Geometry: final body of the model. Coordinates: model frame, mm. A direction names the side the tool comes from. Give positions to 0.01 mm unless a question says otherwise; leave off trailing zeros. Write each loop counter-clockwise with the first axis right and the second up, starting at its lowest first coordinate (ties: lowest second). Pieces come first, ordered by that corner, then holes.
Q1. Section B-B (x = -60). Return the cut outline in (y, z), plus the area to 3 significant figures.
Q2. Section C-C (y = 41). Return the cut outline in (x, z).
Q3. Line query: line 1 (X direction, y = 33.5, z = 1); line 2 (X direction, y = 45.5, z = 9.5); line 3 (X direction, y = 41, z = 9.5). Output: solid intervals per line, ascending.
Q4. Pin query (flat end, axial travel): pin 1 Ø0.6 at (x, z) = (-8.5, 3.5) entering from -Y; pin 2 Ø1.1 at (x, z) = (-26, 4.5) entering from -Y; pin 3 Ø6 at (y, z) = (21.5, 2) entering from +X; pin 4 Ø1 at (x, y) = (-49, 39.5) entering from -Z. Return the tip coordinate at first contact, or that it passes through.
Q5. Section A-A (y = 26). State how many separate pieces and enclosed holes the cut face has, plus the area to 3 significant figures.
Q6. Reachability of faces 4 (the flat face through (-8.34, 38.96, 4.93)), 5 (the flat face through (-24.872, 44, 5)), 6 (the flat face through (-34, 34, 10)) from +Z, -Z, +X, -X, +Y, -Y: full face, straight path, thin tool, end or side. Return the list, or none.
Q7. Mould query, pull axis X, two halves, no side actions, for faces 1 (the cylindrical face through (-44.29, 23.48, 4.93)), 2 (the flat face through (-6.354, 38.929, 4.93)), 3 (the flat face through (-64.68, 48.8, 4.93)). Classes: +X half, -X half, draft (parallel to the pull), parting line (faces both ways), or undercut.
from build123d import *

# Parameters (mm, degrees)
F1_DEPTH = 10


with BuildPart() as f1:
    # F0 (on Top) → F1 (new body)
    with BuildSketch(Plane.XY):
        with BuildLine():
            ThreePointArc((-54.1309299153, 34.7543450507), (-54.1309291616, 34.7521602069), (-54.1309289103, 34.749975363))
            ThreePointArc((-54.1309289103, 34.749975363), (-54.1384443348, 34.3721704089), (-54.1609787174, 33.9949632158))
            ThreePointArc((-54.1609787174, 33.9949632158), (-54.0660685748, 32.5507467457), (-53.7734610387, 31.1333018692))
            ThreePointArc((-53.7734610387, 31.1333018692), (-53.3697669437, 32.5231940325), (-53.1610367081, 33.9553954277))
            ThreePointArc((-53.1610367081, 33.9553954277), (-53.1536089265, 34.335386944), (-53.130987906, 34.7147772626))
            ThreePointArc((-53.130987906, 34.7147772626), (-53.1309436593, 34.7323762881), (-53.1309289103, 34.749975363))
            ThreePointArc((-53.1309289103, 34.749975363), (-53.2282743232, 36.1764316505), (-53.5185055847, 37.5764386092))
            ThreePointArc((-53.5185055847, 37.5764386092), (-53.9221996797, 36.186546446), (-54.1309299153, 34.7543450507))
        make_face()
        with BuildLine():
            ThreePointArc((-54.1609787174, 33.9949632158), (-73.1235001238, 35.1255971916), (-54.1309299153, 34.7543450507))
            ThreePointArc((-54.1309299153, 34.7543450507), (-53.9221996797, 36.186546446), (-53.5185055847, 37.5764386092))
            ThreePointArc((-53.5185055847, 37.5764386092), (-56.911506833, 42.8183932343), (-62.6808702946, 45.2069055352))
            ThreePointArc((-62.6808702946, 45.2069055352), (-63.6810983438, 45.2498555065), (-64.6808702946, 45.1973493436))
            ThreePointArc((-64.6808702946, 45.1973493436), (-71.9280662809, 28.3151085071), (-53.7734610387, 31.1333018692))
            ThreePointArc((-53.7734610387, 31.1333018692), (-54.0660685748, 32.5507467457), (-54.1609787174, 33.9949632158))
        make_face()
        with BuildLine():
            ThreePointArc((-44.6742990635, 44.410760352), (-50.0813318555, 42.2681839255), (-53.5185055847, 37.5764386092))
            ThreePointArc((-53.5185055847, 37.5764386092), (-53.2282743232, 36.1764316505), (-53.1309289103, 34.749975363))
            ThreePointArc((-53.1309289103, 34.749975363), (-53.1309436593, 34.7323762881), (-53.130987906, 34.7147772626))
            ThreePointArc((-53.130987906, 34.7147772626), (-43.3064639701, 43.4531458336), (-34.1611515007, 34.0062619194))
            ThreePointArc((-34.1611515007, 34.0062619194), (-33.9326832198, 35.3653133694), (-33.5195358748, 36.6800482744))
            ThreePointArc((-33.5195358748, 36.6800482744), (-36.8853295304, 41.9809731681), (-42.6742990635, 44.4132978598))
            ThreePointArc((-42.6742990635, 44.4132978598), (-43.674359618, 44.4597566643), (-44.6742990635, 44.410760352))
        make_face()
        with BuildLine():
            ThreePointArc((-53.1610367081, 33.9553954277), (-53.3697669437, 32.5231940325), (-53.7734610387, 31.1333018692))
            ThreePointArc((-53.7734610387, 31.1333018692), (-44.1063222, 23.469211187), (-33.824501511, 30.2865437029))
            ThreePointArc((-33.824501511, 30.2865437029), (-34.1106339928, 31.63463376), (-34.2087077363, 33.0092610331))
            ThreePointArc((-34.2087077363, 33.0092610331), (-44.134704956, 24.4715809191), (-53.1610367081, 33.9553954277))
        make_face()
        with BuildLine():
            ThreePointArc((-64.6808702946, 45.1973493436), (-63.6810983438, 45.2498555065), (-62.6808702946, 45.2069055352))
            Line((-62.6808702946, 45.2069055352), (-62.6808702946, 47.1973493436))
            Line((-62.6808702946, 47.1973493436), (-64.6808702946, 47.1973493436))
            Line((-64.6808702946, 47.1973493436), (-64.6808702946, 45.1973493436))
        make_face()
        with BuildLine():
            Line((-44.6742990635, 46.4132978598), (-44.6742990635, 44.410760352))
            ThreePointArc((-44.6742990635, 44.410760352), (-43.674359618, 44.4597566643), (-42.6742990635, 44.4132978598))
            Line((-42.6742990635, 44.4132978598), (-42.6742990635, 46.4132978598))
            Line((-42.6742990635, 46.4132978598), (-44.6742990635, 46.4132978598))
        make_face()
        with BuildLine():
            ThreePointArc((-34.2087077363, 33.0092610331), (-34.1106339928, 31.63463376), (-33.824501511, 30.2865437029))
            ThreePointArc((-33.824501511, 30.2865437029), (-33.4286074238, 31.6044794904), (-33.2084686098, 32.962870366))
            ThreePointArc((-33.2084686098, 32.962870366), (-33.1985123089, 33.4607100698), (-33.1610380174, 33.9572371849))
            ThreePointArc((-33.1610380174, 33.9572371849), (-33.1610377891, 33.9585011501), (-33.1610377131, 33.9597651154))
            ThreePointArc((-33.1610377131, 33.9597651154), (-33.2510480564, 35.3316672071), (-33.5195358748, 36.6800482744))
            ThreePointArc((-33.5195358748, 36.6800482744), (-33.9326832198, 35.3653133694), (-34.1611515007, 34.0062619194))
            ThreePointArc((-34.1611515007, 34.0062619194), (-34.16106616, 33.983013587), (-34.1610377131, 33.9597651154))
            ThreePointArc((-34.1610377131, 33.9597651154), (-34.1729627034, 33.4839157586), (-34.2087077363, 33.0092610331))
        make_face()
        with BuildLine():
            ThreePointArc((-33.2084686098, 32.962870366), (-33.4286074238, 31.6044794904), (-33.824501511, 30.2865437029))
            ThreePointArc((-33.824501511, 30.2865437029), (-26.0789758688, 23.2083510142), (-16.2744258404, 26.9452986929))
            ThreePointArc((-16.2744258404, 26.9452986929), (-16.2359459807, 28.1016396023), (-16.0452382377, 29.242794962))
            ThreePointArc((-16.0452382377, 29.242794962), (-26.1151867885, 24.2361416337), (-33.2084686098, 32.962870366))
        make_face()
        Polygon((-64.6808702946, 47.1973493436), (-62.6808702946, 47.1973493436), (-61.4884868264, 47.1973493436), (-63.6808702946, 50.3516308963), (-65.7154172659, 47.1973493436), align=None)
        Polygon((-46.2027452886, 46.4132978598), (-44.6742990635, 46.4132978598), (-42.6742990635, 46.4132978598), (-41.1369259803, 46.4132978598), (-43.6742990635, 49.0165157606), align=None)
        with BuildLine():
            ThreePointArc((-16.0452382377, 29.242794962), (-16.2359459807, 28.1016396023), (-16.2744258404, 26.9452986929))
            ThreePointArc((-16.2744258404, 26.9452986929), (-15.6269720373, 27.8983504024), (-15.0934414581, 28.9195502405))
            ThreePointArc((-15.0934414581, 28.9195502405), (-14.849388288, 29.7780382301), (-14.5082524575, 30.6027745052))
            ThreePointArc((-14.5082524575, 30.6027745052), (-14.2932265185, 31.734705525), (-14.2098293285, 32.8838569062))
            ThreePointArc((-14.2098293285, 32.8838569062), (-14.8969732194, 31.9530302459), (-15.4552995863, 30.9396810138))
            ThreePointArc((-15.4552995863, 30.9396810138), (-15.7078230332, 30.0764812725), (-16.0452382377, 29.242794962))
        make_face()
        with BuildLine():
            ThreePointArc((-15.0934414581, 28.9195502405), (-15.6269720373, 27.8983504024), (-16.2744258404, 26.9452986929))
            ThreePointArc((-16.2744258404, 26.9452986929), (-7.3852443737, 18.4842744982), (1.2208400589, 27.2330908929))
            ThreePointArc((1.2208400589, 27.2330908929), (-0.9117259801, 32.9577802096), (-6.269918289, 35.8920059787))
            ThreePointArc((-6.269918289, 35.8920059787), (-7.268206978, 35.9791988017), (-8.269918289, 35.9516789134))
            ThreePointArc((-8.269918289, 35.9516789134), (-11.5444158949, 35.0074217082), (-14.2098293285, 32.8838569062))
            ThreePointArc((-14.2098293285, 32.8838569062), (-14.2932265185, 31.734705525), (-14.5082524575, 30.6027745052))
            ThreePointArc((-14.5082524575, 30.6027745052), (-5.8007888875, 34.7879061456), (0.2208400589, 27.2330908929))
            ThreePointArc((0.2208400589, 27.2330908929), (-8.3774871901, 19.5296604312), (-15.0934414581, 28.9195502405))
        make_face()
        with BuildLine():
            ThreePointArc((-24.8723683958, 43.0098591155), (-30.1154225727, 41.1010441317), (-33.5195358748, 36.6800482744))
            ThreePointArc((-33.5195358748, 36.6800482744), (-33.2510480564, 35.3316672071), (-33.1610377131, 33.9597651154))
            ThreePointArc((-33.1610377131, 33.9597651154), (-33.1610377891, 33.9585011501), (-33.1610380174, 33.9572371849))
            ThreePointArc((-33.1610380174, 33.9572371849), (-23.745452578, 42.0199722388), (-15.2087333715, 33.0319039866))
            ThreePointArc((-15.2087333715, 33.0319039866), (-15.2705874769, 31.9785531588), (-15.4552995863, 30.9396810138))
            ThreePointArc((-15.4552995863, 30.9396810138), (-14.8969732194, 31.9530302459), (-14.2098293285, 32.8838569062))
            ThreePointArc((-14.2098293285, 32.8838569062), (-14.2090073645, 32.9578784182), (-14.2087333715, 33.0319039866))
            ThreePointArc((-14.2087333715, 33.0319039866), (-16.6802799939, 39.6138785947), (-22.8732113197, 42.9423217805))
            ThreePointArc((-22.8732113197, 42.9423217805), (-23.8710969289, 43.0262024429), (-24.8723683958, 43.0098591155))
        make_face()
        with BuildLine():
            Line((-24.8723683958, 45.0098591155), (-24.8723683958, 43.0098591155))
            ThreePointArc((-24.8723683958, 43.0098591155), (-23.8710969289, 43.0262024429), (-22.8732113197, 42.9423217805))
            Line((-22.8732113197, 42.9423217805), (-22.8732113197, 45.0679193003))
            Line((-22.8732113197, 45.0679193003), (-24.8723683958, 45.0098591155))
        make_face()
        with BuildLine():
            ThreePointArc((-8.269918289, 35.9516789134), (-7.268206978, 35.9791988017), (-6.269918289, 35.8920059787))
            Line((-6.269918289, 35.8920059787), (-6.269918289, 37.9516789134))
            Line((-6.269918289, 37.9516789134), (-8.269918289, 37.9516789134))
            Line((-8.269918289, 37.9516789134), (-8.269918289, 35.9516789134))
        make_face()
        Polygon((-26.1985734105, 45.0098591155), (-24.8723683958, 45.0098591155), (-22.8732113197, 45.0679193003), (-21.4801449329, 45.0098591155), (-23.8727898577, 47.6949326694), align=None)
        Polygon((-8.269918289, 37.9516789134), (-6.269918289, 37.9516789134), (-5.4624893661, 37.9516789134), (-7.269918289, 39.9350486696), (-9.4463555142, 37.9516789134), align=None)
    extrude(amount=F1_DEPTH)


solid = f1.part
Computed:
1. outline: (24.9, 0) - (25.97, 0) - (25.97, 10) - (24.9, 10) - close; (43.53, 0) - (44.6, 0) - (44.6, 10) - (43.53, 10) - close
1. area: 21.5 mm2
2. outline: (-72.07, 0) - (-70.79, 0) - (-70.79, 10) - (-72.07, 10) - close; (-56.48, 0) - (-55.19, 0) - (-55.19, 10) - (-56.48, 10) - close; (-51.45, 0) - (-50.04, 0) - (-50.04, 10) - (-51.45, 10) - close; (-37.28, 0) - (-35.87, 0) - (-35.87, 10) - (-37.28, 10) - close; (-30.25, 0) - (-28.39, 0) - (-28.39, 10) - (-30.25, 10) - close; (-20.02, 0) - (-18.17, 0) - (-18.17, 10) - (-20.02, 10) - close
3. line 1: x = -74.06 to -73.05, -54.21 to -53.15, -34.17 to -33.2, -15.22 to -14.22, -13.64 to -12.09, -2.97 to -1.42
3. line 2: x = -64.68 to -62.68, -44.67 to -42.67, -25.77 to -21.92
3. line 3: x = -72.07 to -70.79, -56.48 to -55.19, -51.45 to -50.04, -37.28 to -35.87, -30.25 to -28.39, -20.02 to -18.17
4. pin 1: stops at y = 18.51
4. pin 2: stops at y = 23.11
4. pin 3: stops at x = 0.78
4. pin 4: passes through
5. separate pieces: 8
5. enclosed holes: 0
5. area: 125 mm2
6. face 4: +Z, -Z, +Y
6. face 5: +Z, -Z
6. face 6: +Z, +X, -X, +Y, -Y
7. face 1: undercut
7. face 2: +X half
7. face 3: -X half
